from build123d import *

# Parameters (mm, degrees)
SKETCH_1_R             = 6
SKETCH_1_R_2           = 2.5
EXTRUDE_1_DEPTH        = 19
SKETCH_2_OUTSIDE_W     = 19.096
SKETCH_2_OUTSIDE_H     = 26.096
SKETCH_2_OUTSIDE_R     = 0.75
CUT_EXTRUDE_1_DEPTH    = 9.5
CUT_EXTRUDE_2_DEPTH    = 9.5
HOLE_WIZARD_M4_1_D     = 3.3
HOLE_WIZARD_M4_1_DEPTH = 20
HOLE_WIZARD_M4_1_TIP   = 0.991420021


with BuildPart() as part:
    # 草图1 → 凸台-拉伸1 (new body)
    with BuildSketch(Plane.XY):
        Circle(SKETCH_1_R)
        Circle(SKETCH_1_R_2, mode=Mode.SUBTRACT)
    extrude(amount=EXTRUDE_1_DEPTH)

    # 草图2 outside → 切除-拉伸1 (cut, symmetric)
    with BuildSketch(Plane(origin=(0, 0, 0), x_dir=(1, 0, 0), z_dir=(0, 1, 0))):
        with Locations((0, -9.5)):
            Rectangle(SKETCH_2_OUTSIDE_W, SKETCH_2_OUTSIDE_H)
        with BuildLine():
            Line((-2.75, -2.75), (-2.75, -9))
            ThreePointArc((-2.75, -9), (-3.701902961, -11.298097039), (-6, -12.25))
            Line((-6, -12.25), (-6, -19))
            Line((-6, -19), (6, -19))
            Line((6, -19), (6, -12.25))
            ThreePointArc((6, -12.25), (3.701902961, -11.298097039), (2.75, -9))
            Line((2.75, -9), (2.75, -2.75))
            ThreePointArc((2.75, -2.75), (0, 0), (-2.75, -2.75))
        make_face(mode=Mode.SUBTRACT)
        with Locations((0, -2.75)):
            Circle(SKETCH_2_OUTSIDE_R)
    extrude(amount=CUT_EXTRUDE_1_DEPTH, both=True, mode=Mode.SUBTRACT)

    # 草图3 → 切除-拉伸2 (cut, symmetric)
    with BuildSketch(Plane(origin=(0, 0, 0), x_dir=(0, 0, -1), z_dir=(1, 0, 0))):
        with BuildLine():
            Line((-9.250000001, 3), (0, 3))
            Line((0, 3), (0, -3))
            Line((0, -3), (-9.250000001, -3))
            ThreePointArc((-9.250000001, -3), (-12.250000001, 0), (-9.250000001, 3))
        make_face()
    extrude(amount=CUT_EXTRUDE_2_DEPTH, both=True, mode=Mode.SUBTRACT)

    # M4 螺纹孔1
    with Locations(Plane(origin=(0, 6, 0), x_dir=(1, 0, 0), z_dir=(0, 1, 0))):
        with Locations((0, -15.5)):
            Hole(HOLE_WIZARD_M4_1_D / 2, depth=HOLE_WIZARD_M4_1_DEPTH)
            with Locations((0, 0, -(HOLE_WIZARD_M4_1_DEPTH + HOLE_WIZARD_M4_1_TIP / 2))):  # 118° drill point
                Cone(0, HOLE_WIZARD_M4_1_D / 2, HOLE_WIZARD_M4_1_TIP, mode=Mode.SUBTRACT)


solid = part.part
The listing builds one solid part. Answer for the finished solid, in the listing's coordinates (mm). A direction names the side the tool comes from. Coordinates: 2 decimals unless noted, no trailing zeros. Loops run counter-clockwise (first coordinate to the right, second up) from the corner with the lowest first, then second, coordinate; pieces in that order, holes last.
1) Find section C-C on z = 2.25. Write down the section's boundary in (x, y).
2) A tool of negligible diameter and unlimited length cuts with its end or side. For faces 1 (the face through (0, -4, 2)), 2 (the face through (2.75, 4, 6)), 3 (the face through (0, 3, 5)), from which of +Z, -Z, +X, -X, +Y, -Y can it reach the whole face along a straight path? Write none if from no direction.
3) Find section B-B on y = 3.75. Write down the section's boundary in (x, z).
4) Flat-ended cylindrical pins translate along their axes: pin 1 Ø1.2 at (x, z) = (0, 2.75) entering from -Y; pin 2 Ø1.5 at (x, y) = (-3, -4.5) entering from -Z; pin 3 Ø2.5 at (y, z) = (-4, 5.5) entering from -X; pin 4 Ø5 at (x, z) = (-4, 7) entering from -Y. Find the tip coordinate at first contact, or state that the pin passes through.
5) Find the intervals of material crossed by L1, parallel to Z at x = 0, y = 3.85; L2, parallel to X at y = -3.65, z = 2.75; L3, parallel to Y at x = -0.25, z = 5, in increasing order.
6) Determine the mould class of faces 4 (the face through (-2.75, 4, 6)), 5 (the face through (0, 4, 0)), 6 (the face through (2.31, -0.96, 14.9)), 7 (the face through (1.31, -3.97, 16.5)) for opening direction X: pulls with the +X half, pulls with the -X half, needs draft (parallel to the pull), parting line crosses it, or undercut.
7) Find section D-D on y = -1. Write down the section's boundary in (x, z), then the cut area to 3 significant figures.
8) Find section A-A on x = 0. Write down the section's boundary in (y, z).
Values:
1. outline: (-2.7, -5.36) arc R6 ccw to (-0.56, -5.97) - (-0.56, -3) - (-2.7, -3) - close; (-2.7, 3) - (-0.56, 3) - (-0.56, 5.97) arc R6 ccw to (-2.7, 5.36) - close; (0.56, -5.97) arc R6 ccw to (2.7, -5.36) - (2.7, -3) - (0.56, -3) - close; (0.56, 3) - (2.7, 3) - (2.7, 5.36) arc R6 ccw to (0.56, 5.97) - close
2. face 1: +Y, -Y
2. face 2: -Z, +X, +Y, -Y
2. face 3: -Z, +X, -X
3. outline: (-4.68, 11.97) arc R3.25 cw to (-2.75, 9) - (-2.75, 2.75) arc R2.75 ccw to (2.75, 2.75) - (2.75, 9) arc R3.25 cw to (4.68, 11.97) - (4.68, 19) - (-4.68, 19) - close; hole circle Ø3.3 at (0, 15.5); hole circle Ø1.5 at (0, 2.75)
4. pin 1: passes through
4. pin 2: stops at z = 1.17
4. pin 3: stops at x = -2.75
4. pin 4: stops at y = -5.81
5. L1: z = 0 to 2, 3.5 to 13.85, 17.15 to 19
5. L2: x = -2.75 to -0.75, 0.75 to 2.75
5. L3: y = -5.99 to -3, 3 to 5.99
6. face 4: pulls with the -X half
6. face 5: parting line crosses it
6. face 6: undercut
6. face 7: undercut
7. outline: (-5.92, 12.25) arc R3.25 cw to (-4.96, 12.08) - (-2.29, 12.08) - (-2.29, 19) - (-5.92, 19) - close; (2.29, 12.08) - (4.96, 12.08) arc R3.25 cw to (5.92, 12.25) - (5.92, 19) - (2.29, 19) - close
7. area: 50.0 mm2
8. outline: (-6, 0) - (-3, 0) - (-3, 2) - (-6, 2) - close; (-6, 3.5) - (-3, 3.5) - (-3, 9.25) arc R3 cw to (-2.5, 10.91) - (-2.5, 13.85) - (-6, 13.85) - close; (-6, 17.15) - (-2.5, 17.15) - (-2.5, 19) - (-6, 19) - close; (2.5, 10.91) arc R3 cw to (3, 9.25) - (3, 3.5) - (6, 3.5) - (6, 13.85) - (2.5, 13.85) - close; (2.5, 17.15) - (6, 17.15) - (6, 19) - (2.5, 19) - close; (3, 0) - (6, 0) - (6, 2) - (3, 2) - close
